```python
from build123d import *

# Parameters (mm, degrees)
F1_DEPTH = 25.4
F3_DEPTH = 50.801
F5_DEPTH = 12.701
F7_DEPTH = 25.4


with BuildPart() as f1:
    # F0 (on Front) → F1 (new body)
    with BuildSketch(Plane.XZ):
        Polygon((0, 12.7), (0, 0), (76.2, 0), (76.2, 12.7), (50.8, 12.7), (50.8, 44.45), (25.4, 44.45), (25.4, 12.7), align=None)
    extrude(amount=F1_DEPTH)

    # F2 (on face) → F3 (cut, through all)
    with BuildSketch(Plane.YZ.offset(50.8)):
        with BuildLine():
            Line((-19.05, 28.575), (-6.35, 28.575))
            ThreePointArc((-6.35, 28.575), (-12.7, 34.925), (-19.05, 28.575))
        make_face()
        with BuildLine():
            ThreePointArc((-19.05, 28.575), (-12.7, 22.225), (-6.35, 28.575))
            Line((-6.35, 28.575), (-19.05, 28.575))
        make_face()
        with BuildLine():
            ThreePointArc((-25.4, 28.575), (-12.7, 41.275), (0, 28.575))
            Line((0, 28.575), (0, 44.45))
            Line((0, 44.45), (-25.4, 44.45))
            Line((-25.4, 44.45), (-25.4, 28.575))
        make_face()
    extrude(amount=-F3_DEPTH, mode=Mode.SUBTRACT)

    # F4 (on face) → F5 (cut, through all)
    with BuildSketch(Plane.XY.offset(12.7)):
        with BuildLine():
            ThreePointArc((12.7, -6.35), (6.35, -12.7), (12.7, -19.05))
            Line((12.7, -19.05), (12.7, -6.35))
        make_face()
        with BuildLine():
            Line((12.7, -6.35), (12.7, -19.05))
            ThreePointArc((12.7, -19.05), (17.1901280605, -17.1901280605), (19.05, -12.7))
            ThreePointArc((19.05, -12.7), (17.1901280605, -8.2098719395), (12.7, -6.35))
        make_face()
        with BuildLine():
            Line((0, 0), (0, -12.7))
            ThreePointArc((0, -12.7), (3.7197438789, -3.7197438789), (12.7, 0))
            Line((12.7, 0), (0, 0))
        make_face()
        with BuildLine():
            Line((0, -25.4), (12.7, -25.4))
            ThreePointArc((12.7, -25.4), (3.7197438789, -21.6802561211), (0, -12.7))
            Line((0, -12.7), (0, -25.4))
        make_face()
    extrude(amount=-F5_DEPTH, mode=Mode.SUBTRACT)

    # F6 (on face) → F7 (cut)
    with BuildSketch(Plane.XY.offset(12.7)):
        with BuildLine():
            Line((63.5, -19.05), (63.5, -6.35))
            ThreePointArc((63.5, -6.35), (57.15, -12.7), (63.5, -19.05))
        make_face()
        with BuildLine():
            ThreePointArc((69.85, -12.7), (67.9901280605, -8.2098719395), (63.5, -6.35))
            Line((63.5, -6.35), (63.5, -19.05))
            ThreePointArc((63.5, -19.05), (67.9901280605, -17.1901280605), (69.85, -12.7))
        make_face()
        with BuildLine():
            Line((76.2, 0), (63.5, 0))
            ThreePointArc((63.5, 0), (72.4802561211, -3.7197438789), (76.2, -12.7))
            Line((76.2, -12.7), (76.2, 0))
        make_face()
        with BuildLine():
            Line((76.2, -25.4), (76.2, -12.7))
            ThreePointArc((76.2, -12.7), (72.4802561211, -21.6802561211), (63.5, -25.4))
            Line((63.5, -25.4), (76.2, -25.4))
        make_face()
    extrude(amount=-F7_DEPTH, mode=Mode.SUBTRACT)


solid = f1.part
```
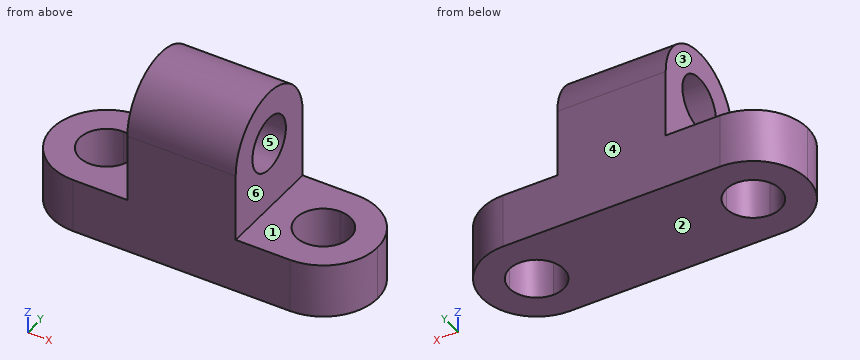
Input: part model. Units: mm. Frame: model coordinates. Face numbers are marked on the shaded views. A direction names the side the tool comes from. Give positions to 0.01 mm unless a question says otherwise; leave off trailing zeros. Order: outer loops, then holes, each group sorted by start corner. A loop starts at its lowest first (then second) coordinate and runs counter-clockwise, first axis right, second up. Notation, with made-up numbers: (66.5, 20) -> (84.5, 20) arc R23 ccw to (84.5, 32) -> close; hole circle Ø3 at (74.25, 61). An arc over 180 degrees is marked (long way). Write each question's results on one line, items separated by ' | '. Start each with the question number.
Item 1: Set-up query: the marked faces 1, 2 and 3. Return all of +Z, -Z, +X, -X, +Y, -Y with unobstructed straight access to the full face (end or side cutting, diameter ignored); none if empty.
Item 2: Line query: line 1 (Z direction, x = 45.5, y = -12.7) (3 decimals); line 2 (X direction, y = -15.5, z = 9.5); line 3 (X direction, y = -18.25, z = 9). Output: solid intervals per line, ascending.
Item 3: Contact query for flat-ended pins moving along their axis: P1, Ø7.5, axis at x = 12.5, y = -10, coming from the +Z side; P2, Ø12, axis at y = -19, z = 8, coming from the +X side; P3, Ø1.5, axis at y = -6, z = 13, coming from the -X side. Output: stop coordinate, or through.
Item 4: Cut plane D-D on y = -1.5. Return the cut outline in (x, z), then the cut area to 3 significant figures.
Item 5: Mould query, pull axis Y, two halves, no side actions, for the marked faces 4, 5 and 6. Classes: pulls with the +Y half, pulls with the -Y half, needs draft (parallel to the pull), parting line crosses it, or undercut.
Item 6: Cut plane A-A on z = 7. Return the cut outline in (x, y), then the cut area to 3 significant figures.
Item 7: Cut plane C-C on x = 32. Return the cut outline in (y, z) (3 decimals), then the cut area to 3 significant figures.
Item 8: Cut plane B-B on y = -8.25. Return the cut outline in (x, z), then the cut area to 3 significant figures.
Established:
1) face 1: +Z, +X, +Y, -Y | face 2: -Z, +X, -X, +Y, -Y | face 3: +Z, -X, +Y, -Y
2) line 1: 0 to 22.225, 34.925 to 41.275 | line 2: 0.31 to 7, 18.4 to 57.8, 69.2 to 75.89 | line 3: 1.28 to 9.61, 15.79 to 60.41, 66.59 to 74.92
3) P1: z = 12.7 | P2: x = 76.2 | P3: x = 1.51
4) outline: (6.71, 0) -> (69.49, 0) -> (69.49, 12.7) -> (50.8, 12.7) -> (50.8, 34.56) -> (25.4, 34.56) -> (25.4, 12.7) -> (6.71, 12.7) -> close | area: 1,350 mm^2
5) face 4: pulls with the +Y half | face 5: undercut | face 6: needs draft
6) outline: (12.7, -25.4) -> (63.5, -25.4) arc R12.7 ccw to (63.5, 0) -> (12.7, 0) arc R12.7 ccw to start; hole circle Ø12.7 at (12.7, -12.7); hole circle Ø12.7 at (63.5, -12.7) | area: 1,540 mm^2
7) outline: (-25.4, 0) -> (0, 0) -> (0, 28.575) arc R12.7 ccw to (-25.4, 28.575) -> close; hole circle Ø12.7 at (-12.7, 28.575) | area: 852 mm^2
8) outline: (0.81, 0) -> (8.17, 0) -> (8.17, 12.7) -> (0.81, 12.7) -> close; (17.23, 0) -> (58.97, 0) -> (58.97, 12.7) -> (50.8, 12.7) -> (50.8, 24.05) -> (25.4, 24.05) -> (25.4, 12.7) -> (17.23, 12.7) -> close; (25.4, 33.1) -> (50.8, 33.1) -> (50.8, 40.47) -> (25.4, 40.47) -> close; (68.03, 0) -> (75.39, 0) -> (75.39, 12.7) -> (68.03, 12.7) -> close | area: 1,190 mm^2
